The model under review builds one solid part; all positions refer to its coordinate system, in mm. A direction names the side the tool comes from. Give positions to 0.01 mm unless a question says otherwise; leave off trailing zeros. Loops run counter-clockwise (first coordinate to the right, second up) from the corner with the lowest first, then second, coordinate; pieces in that order, holes last. Notation, with made-up numbers: (69.25, -36) - (107.25, -36) arc R20 ccw to (107.25, -13) - close; hole circle Ø9 at (21, 13.5). An arc over 180 degrees is marked (long way). Answer as a JSON object with one key per item and string values.
from build123d import *

# Parameters (mm, degrees)
SKETCH1_W           = 45
SKETCH1_H           = 60
BOSS_EXTRUDE1_DEPTH = 157
SKETCH2_W           = 6
SKETCH2_H           = 15
BOSS_EXTRUDE2_DEPTH = 15
FILLET1_R           = 2.5


with BuildPart() as part:
    # Sketch1 → Boss-Extrude1 (new body)
    with BuildSketch(Plane(origin=(0, 0, 0), x_dir=(1, 0, 0), z_dir=(0, 1, 0))):
        with Locations((22.5, 30)):
            Rectangle(SKETCH1_W, SKETCH1_H)
    extrude(amount=BOSS_EXTRUDE1_DEPTH)

    # Sketch2 → Boss-Extrude2 (add)
    with BuildSketch(Plane(origin=(0, 157, 0), x_dir=(1, 0, 0), z_dir=(0, 1, 0))):
        with Locations((42, 30)):
            Rectangle(SKETCH2_W, SKETCH2_H)
    extrude(amount=BOSS_EXTRUDE2_DEPTH)

    # Fillet1
    fillet1_edges = [part.edges().sort_by_distance(p)[0] for p in [
        (45, 157, -11.25),
        (45, 157, -48.75),
        (45, 164.5, -22.5),
        (45, 164.5, -37.5),
        (22.5, 157, -60),
        (45, 172, -30),
        (0, 157, -30),
        (22.5, 0, -60),
        (45, 0, -30),
        (22.5, 0, 0),
        (0, 0, -30),
        (0, 78.5, -60),
        (45, 78.5, -60),
        (45, 78.5, 0),
        (0, 78.5, 0),
        (22.5, 157, 0),
    ]]
    fillet(fillet1_edges, radius=FILLET1_R)


solid = part.part
Q1. Consider section B-B, the plane x = 26. State the section outline as (y, z) points.
Results:
{"outline": "(0, -57.5) arc R2.5 ccw to (2.5, -60) - (154.5, -60) arc R2.5 ccw to (157, -57.5) - (157, -2.5) arc R2.5 ccw to (154.5, 0) - (2.5, 0) arc R2.5 ccw to (0, -2.5) - close"}
Q2. For faces 1 (the face through (41, 164, -37.5)), 2 (the face through (39, 164, -30)), 3 (the face through (22, 77, -60)), 4 (the face through (41, 164, -22.5)), list the 3-axis set-ups (+Z, -Z, +X, -X, +Y, -Y) from which the entire face can be reached by the end or side of a thin tool; tool diameter is ignored.
Results:
{"face 1": "-Z, +X, -X, +Y", "face 2": "+Z, -Z, -X, +Y", "face 3": "-Z, +X, -X, +Y, -Y", "face 4": "+Z, +X, -X, +Y"}
Q3. Consider section D-D, the plane z = -33. State the section outline as (x, y) points, plus the area to 3 significant figures.
Results:
{"outline": "(0, 2.5) arc R2.5 ccw to (2.5, 0) - (42.5, 0) arc R2.5 ccw to (45, 2.5) - (45, 169.5) arc R2.5 ccw to (42.5, 172) - (39, 172) - (39, 157) - (2.5, 157) arc R2.5 ccw to (0, 154.5) - close", "area": "7,150 mm^2"}
Q4. Consider section A-A, the plane z = -49. State the section outline as (x, y) points, plus the area to 3 significant figures.
Results:
{"outline": "(0, 2.5) arc R2.5 ccw to (2.5, 0) - (42.5, 0) arc R2.5 ccw to (45, 2.5) - (45, 154.5) arc R2.5 ccw to (42.5, 157) - (2.5, 157) arc R2.5 ccw to (0, 154.5) - close", "area": "7,060 mm^2"}
Q5. Consider section C-C, the plane y = 159.5. State the section outline as (x, z) points, plus the area to 3 significant figures.
Results:
{"outline": "(39, -37.5) - (42.5, -37.5) arc R2.5 ccw to (45, -35) - (45, -25) arc R2.5 ccw to (42.5, -22.5) - (39, -22.5) - close", "area": "87.3 mm^2"}
Q6. Clearance check with flat-ended pins moving along their axes: pin 1 Ø1 at (x, y) = (41.5, 162) entering from +Z; pin 2 Ø10 at (x, z) = (15, -22.5) entering from +Y; pin 3 Ø1.8 at (x, y) = (40.5, 166.5) entering from -Z; pin 4 Ø6 at (y, z) = (48, -28.5) entering from -X. State where each tip first meets the part, or that it passes through.
Results:
{"pin 1": "stops at z = -22.5", "pin 2": "stops at y = 157", "pin 3": "stops at z = -37.5", "pin 4": "stops at x = 0"}
Q7. To check wall thickness, follow probe 1 along Y at (x, z) = (28, -42). State the ranges of the line that lie inside material, in increasing order. Write a range as [from, to].
Results:
{"probe 1": "y = [0, 157]"}
